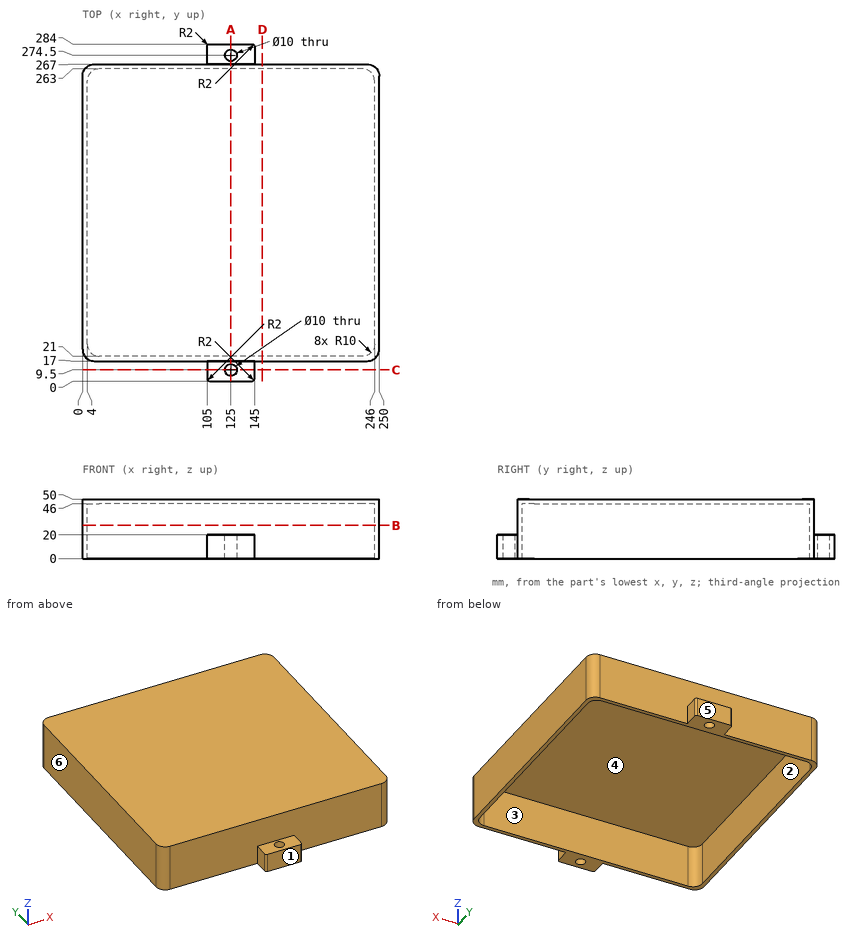
Can you work these out from the drawing? Everything is in mm from the part's minimum corner. A direction names the side the tool comes from. Round coordinates to 2 decimals unless told otherwise and drop trailing zeros. Order: outer loops, then holes, each group sorted by start corner. A loop starts at its lowest first (then second) coordinate and runs counter-clockwise, first axis right, second up. Notation, with made-up numbers: (29.25, 10) -> (65.25, 10) arc R26 ccw to (65.25, 31) -> close; hole circle Ø5 at (-11.5, -37.5). An arc over 180 degrees is marked (long way). Use CSV: the item, a comma, the result in double quotes.
1. I want a section at D-D on x = 151.5. List the corners of the cut face in (y, z) for me, and give its area (3 significant figures).
Recorded:
outline,"(17, 0) -> (21, 0) -> (21, 46) -> (263, 46) -> (263, 0) -> (267, 0) -> (267, 50) -> (17, 50) -> close"
area,"1,370 mm2"
2. Thinking about a two-plate mould opening in X: for the marked faces 3, 4, 5 and 6, which applies, pulls with the +X half, pulls with the -X half, needs draft (parallel to the pull), parting line crosses it, or undercut?
Recorded:
face 3,"undercut"
face 4,"undercut"
face 5,"needs draft"
face 6,"pulls with the -X half"
3. I want a section at A-A on x = 125. List the corners of the cut face in (y, z) for me.
Recorded:
outline,"(0, 0) -> (4.5, 0) -> (4.5, 20) -> (0, 20) -> close; (14.5, 0) -> (21, 0) -> (21, 46) -> (263, 46) -> (263, 0) -> (269.5, 0) -> (269.5, 20) -> (267, 20) -> (267, 50) -> (17, 50) -> (17, 20) -> (14.5, 20) -> close; (279.5, 0) -> (284, 0) -> (284, 20) -> (279.5, 20) -> close"
4. I'm going to push flat-ended pins straight in: P1, Ø5, axis at x = 133.5, y = 271.5, coming from the +Z side; P2, Ø10, axis at x = 69, z = 38, coming from the -Y side; P3, Ø4.5, axis at y = 12, z = 6, coming from the +X side. Where does each tip first touch, or does it pass through?
Recorded:
P1,"stops at z = 20"
P2,"stops at y = 17"
P3,"stops at x = 145"
5. I need wall thicknesses on line 1 along Y through (x, z) = (125, 6.75); line 2 along Y through (x, z) = (13.5, 34); line 3 along X through (y, z) = (81, 33). Which ranges of each line are inside material? Lowest first, please.
Recorded:
line 1,"y = 0 to 4.5, 14.5 to 21, 263 to 269.5, 279.5 to 284"
line 2,"y = 17 to 21.01, 262.99 to 267"
line 3,"x = 0 to 4, 246 to 250"
6. I want a section at C-C on y = 9.5. List the corners of the cut face in (x, z) for me, and give its area (3 significant figures).
Recorded:
outline,"(105, 0) -> (120, 0) -> (120, 20) -> (105, 20) -> close; (130, 0) -> (145, 0) -> (145, 20) -> (130, 20) -> close"
area,"600 mm2"
7. Which directions (+Z, -Z, +X, -X, +Y, -Y) give clear straight access to the entire face, cutting with the end or side of a thin tool? Please do the marked faces 1 and 2.
Recorded:
face 1,"+Z, -Z, +X, -X, -Y"
face 2,"-Z"
8. I want a section at B-B on z = 28. List the corners of the cut face in (x, y) for me.
Recorded:
outline,"(0, 27) arc R10 ccw to (10, 17) -> (240, 17) arc R10 ccw to (250, 27) -> (250, 257) arc R10 ccw to (240, 267) -> (10, 267) arc R10 ccw to (0, 257) -> close; hole (4, 31) arc R10 ccw to (14, 21) -> (236, 21) arc R10 ccw to (246, 31) -> (246, 253) arc R10 ccw to (236, 263) -> (14, 263) arc R10 ccw to (4, 253) -> close"
